from build123d import *

# Parameters (mm, degrees)
F_9_0_9_DIAMETER_HOLE1_D     = 9
CUT_EXTRUDE1_DEPTH           = 31.070749908
CUT_EXTRUDE1_DEPTH_BACK      = 1.5
SKETCH6_R                    = 5.75
CUT_EXTRUDE2_START           = -12
SKETCH6_2_R                  = 5.75
CUT_EXTRUDE2_DEPTH           = 1.5
BOSS_EXTRUDE1_START          = -10.5
BOSS_EXTRUDE1_DEPTH          = 10.5
TAP_DRILL_FOR_M3_HELICOIL1_D = 3.15
SKETCH11_R                   = 19
SKETCH11_R_2                 = 17
CUT_EXTRUDE3_DEPTH           = 1.5


with BuildPart() as part:
    # Sketch1 → Revolve1 (revolve)
    with BuildSketch(Plane.XY, mode=Mode.PRIVATE) as revolve1_sk:
        Polygon((0, 0), (19, 0), (19, 3.5), (17.5, 3.5), (17.5, 10), (19, 10), (19, 13.5), (0, 13.5), align=None)
    revolve(revolve1_sk.sketch.rotate(Axis((0, 13.5, 0), (0, -1, 0)), 90), axis=Axis((0, 13.5, 0), (0, -1, 0)))

    # Ø9.0 (9) Diameter Hole1 (through all)
    with Locations(Plane(origin=(0, 13.5, 0), x_dir=(1, 0, 0), z_dir=(0, 1, 0))):
        with Locations((0, 0)):
            Hole(F_9_0_9_DIAMETER_HOLE1_D / 2)

    # Sketch6 → Cut-Extrude1 (cut, two sides: drawn at the far end of the back side and taken through both)
    with BuildSketch(Plane(origin=(0, 13.5, 0), x_dir=(1, 0, 0), z_dir=(0, 1, 0)).offset(-CUT_EXTRUDE1_DEPTH_BACK)):
        with Locations(Location((0, 0, 0), (0, 0, 90))):
            Circle(SKETCH6_R)
    extrude(amount=CUT_EXTRUDE1_DEPTH + CUT_EXTRUDE1_DEPTH_BACK, mode=Mode.SUBTRACT)

    # Sketch6<2> → Cut-Extrude2 (cut)
    with BuildSketch(Plane(origin=(0, 13.5, 0), x_dir=(1, 0, 0), z_dir=(0, 1, 0)).offset(CUT_EXTRUDE2_START)):
        with Locations(Location((0, 0, 0), (0, 0, 90))):
            Circle(SKETCH6_2_R)
    extrude(amount=-CUT_EXTRUDE2_DEPTH, mode=Mode.SUBTRACT)

    # Sketch7 → Boss-Extrude1 (add)
    with BuildSketch(Plane(origin=(0, 12, 0), x_dir=(1, 0, 0), z_dir=(0, 1, 0)).offset(BOSS_EXTRUDE1_START)):
        with BuildLine():
            ThreePointArc((-4, 2.061552813), (-4.5, 0), (-4, -2.061552813))
            Line((-4, -2.061552813), (-4, 2.061552813))
        make_face()
        with BuildLine():
            Line((4, 2.061552813), (4, -2.061552813))
            ThreePointArc((4, -2.061552813), (4.373213921, -1.060660172), (4.5, 0))
            ThreePointArc((4.5, 0), (4.373213921, 1.060660172), (4, 2.061552813))
        make_face()
    extrude(amount=BOSS_EXTRUDE1_DEPTH)

    # Tap Drill for M3 Helicoil1 (through all)
    with Locations(Plane(origin=(0, 13.5, 0), x_dir=(1, 0, 0), z_dir=(0, 1, 0))):
        with Locations((-11.888206454, 3.86271243), (0, 12.5), (11.888206454, 3.86271243), (7.347315654, -10.11271243), (-7.347315654, -10.11271243)):
            Hole(TAP_DRILL_FOR_M3_HELICOIL1_D / 2)

    # Sketch11 → Cut-Extrude3 (cut)
    with BuildSketch(Plane(origin=(0, 13.5, 0), x_dir=(1, 0, 0), z_dir=(0, 1, 0))):
        with Locations(Location((0, 0, 0), (0, 0, 270))):
            Circle(SKETCH11_R)
        with Locations(Location((0, 0, 0), (0, 0, 270))):
            Circle(SKETCH11_R_2, mode=Mode.SUBTRACT)
    extrude(amount=-CUT_EXTRUDE3_DEPTH, mode=Mode.SUBTRACT)


solid = part.part
Can you work these out from the model? Positions are in its coordinate system, mm. A direction names the side the tool comes from. Give positions to 0.01 mm unless a question says otherwise; leave off trailing zeros. Loops run counter-clockwise (first coordinate to the right, second up) from the corner with the lowest first, then second, coordinate; pieces in that order, holes last. Notation, with made-up numbers: (34, -39.75) -> (71, -39.75) arc R12 ccw to (71, -20.75) -> close; hole circle Ø1 at (79, 68.5). An arc over 180 degrees is marked (long way). Use one line per item in the form item = value.
1) If we section it at D-D (z = 8): Please give me the cut outline in (x, y).
Answers:
outline = (-17.23, 0) -> (17.23, 0) -> (17.23, 3.5) -> (15.56, 3.5) -> (15.56, 10) -> (17.23, 10) -> (17.23, 12) -> (15, 12) -> (15, 13.5) -> (-15, 13.5) -> (-15, 12) -> (-17.23, 12) -> (-17.23, 10) -> (-15.56, 10) -> (-15.56, 3.5) -> (-17.23, 3.5) -> close
2) If we section it at B-B (x = 7.5): Please give me the cut outline in (y, z).
Answers:
outline = (0, -17.46) -> (3.5, -17.46) -> (3.5, -15.81) -> (10, -15.81) -> (10, -17.46) -> (12, -17.46) -> (12, -15.26) -> (13.5, -15.26) -> (13.5, 8.55) -> (0, 8.55) -> close; (0, 11.68) -> (13.5, 11.68) -> (13.5, 15.26) -> (12, 15.26) -> (12, 17.46) -> (10, 17.46) -> (10, 15.81) -> (3.5, 15.81) -> (3.5, 17.46) -> (0, 17.46) -> close
3) For faces 5 (the face through (6, 3.5, 17)), 6 (the face through (4.2, 12, 0.4)), 7 (the face through (-0.1, 6.7, -4.5)), which set-ups out of +Z, -Z, +X, -X, +Y, -Y let a thin tool reach every point of the face, with its end or its side?
Answers:
face_5 = none
face_6 = +Y
face_7 = +Y, -Y
4) We'd pull the mould along X, two halves only. Please class faces 1 (the face through (7, 13.5, 0)), 2 (the face through (18.548, 11.014, -4.119)), 3 (the face through (4.2, 1.5, 0.4)), 4 (the face through (0.21, 6.66, -14.06)): released by +X, released by -X, zero draft, split by the parting line, or undercut.
Answers:
face_1 = zero draft
face_2 = split by the parting line
face_3 = undercut
face_4 = undercut
5) I need wall thicknesses on line 1 along Y through (x, z) = (-14.5, 10.5); line 2 along X through (y, z) = (12.85, 0); line 3 along X through (y, z) = (3, -5). Which ranges of each line are inside material? Lowest first, please.
Answers:
line_1 = 0 to 3.5, 10 to 12
line_2 = -17 to -5.75, 5.75 to 17
line_3 = -18.33 to -12.98, -10.8 to 10.8, 12.98 to 18.33
6) If we section it at A-A (z = 0): Please give me the cut outline in (x, y).
Answers:
outline = (-19, 0) -> (-5.75, 0) -> (-5.75, 1.5) -> (-4, 1.5) -> (-4, 12) -> (-5.75, 12) -> (-5.75, 13.5) -> (-17, 13.5) -> (-17, 12) -> (-19, 12) -> (-19, 10) -> (-17.5, 10) -> (-17.5, 3.5) -> (-19, 3.5) -> close; (4, 1.5) -> (5.75, 1.5) -> (5.75, 0) -> (19, 0) -> (19, 3.5) -> (17.5, 3.5) -> (17.5, 10) -> (19, 10) -> (19, 12) -> (17, 12) -> (17, 13.5) -> (5.75, 13.5) -> (5.75, 12) -> (4, 12) -> close
7) If we section it at C-C (y = 8): Please give me the cut outline in (x, z) (3 decimals).
Answers:
outline = circle Ø35 at (0, 0); hole circle Ø3.15 at (-11.888, -3.863); hole circle Ø3.15 at (-7.347, 10.113); hole (-4, -2.062) arc R4.5 ccw to (4, -2.062) -> (4, 2.062) arc R4.5 ccw to (-4, 2.062) -> close; hole circle Ø3.15 at (0, -12.5); hole circle Ø3.15 at (7.347, 10.113); hole circle Ø3.15 at (11.888, -3.863)
8) Will these pins go through, and if not, where does the flat tip stop? pin 1 (1.5 mm diameter, centred on x = 2, y = 10, fed in from -Z); pin 2 (3 mm diameter, centred on x = -7.35, z = 10.11, fed in from +Y); pin 3 (1.5 mm diameter, centred on y = 4.5, z = 5, fed in from +X); pin 4 (3.5 mm diameter, centred on y = 7, z = 0, fed in from -X).
Answers:
pin_1 = -18.96
pin_2 = through
pin_3 = 16.98
pin_4 = -17.5
